Input: part model. Units: mm. Frame: model coordinates. A direction names the side the tool comes from. Give positions to 0.01 mm unless a question says otherwise; leave off trailing zeros. Loops run counter-clockwise (first coordinate to the right, second up) from the corner with the lowest first, then second, coordinate; pieces in that order, holes last. Notation, with made-up numbers: M 75,82.5 L 106,82.5 A6 cw 106,91.5 Z; hole C 83,-1 d3. An arc over 180 degrees is marked long. Answer as a JSON object with one key per item and string values. Group by question number.
1) Draft query along X for faces 1 (the flat face through (18.7, -1, 3)), 2 (the flat face through (14, 8, 0)), 3 (the flat face through (12, 9, -3)), 4 (the flat face through (25.7, 1, 2)). Return one class per face: +X half, -X half, draft (parallel to the pull), parting line (faces both ways), or undercut.
2) Section query A-A on y = 15.75. Return loops of the section in (x, z).
3) Section query B-B on x = 16.75. Return loops of the section in (y, z), plus the area to 4 significant figures.
4) First-contact query: P1, Ø0.9, axis at y = 10.5, z = -1, coming from the +X side; P2, Ø6, axis at x = 15.5, y = 9, coming from the +Z side. Flat tips, straight axial feed; report the tip coordinate or a pass-through.
5) Access query for faces 5 (the flat face through (23.7, 9, -1)), 6 (the flat face through (17.7, 17, -1)), 7 (the flat face through (12.7, -1, 3)), 8 (the flat face through (23.7, 2, 3)). Directions: +Z, -Z, +X, -X, +Y, -Y. A direction counts if a zero-diameter tool reaches every point of the face in a straight line with its end or side. Return the directions, or none.
6) Ray query, L1, parallel to Y at x = 7, z = -1.75; L2, parallel to Y at x = 2.5, z = 2.25; L3, parallel to X at y = 14.75, z = 0.5. Return the intervals inside material, ascending.
7) Section query D-D on z = -2. Return loops of the section in (x, y).
8) Section query C-C on z = 3.25. Return loops of the section in (x, y).
Autodesk Fusion 360 part; units mm, degrees
sketch "Sketch1" plane through (0, 0, 0) normal (0, 0, 1) x (1, 0, 0) in component "case"
  line L0 (0, 0) -> (23.7, 0)
  line L1 (23.7, 0) -> (23.7, 18.6)
  line L2 (23.7, 18.6) -> (0, 18.6)
  line L3 (0, 18.6) -> (0, 0)
  circle A0 centre (21, 16.05) radius 1.5
  circle A1 centre (21, 2.55) radius 1.5
  line L4 (21, 16.05) -> (21, 2.55) construction
  line L5 (23.7, 9.3) -> (0, 9.3) construction
  line L6 (3.75, 0) -> (3.75, 14.85)
  line L7 (3.75, 14.85) -> (17.7, 14.85)
  line L8 (17.7, 14.85) -> (17.7, 18.6)
  line L9 (-2, 21.6) -> (25.7, 21.6)
  line L10 (25.7, 21.6) -> (25.7, -3)
  line L11 (25.7, -3) -> (-2, -3)
  line L12 (-2, -3) -> (-2, 21.6)
  line L13 (11.85, -3) -> (11.85, 21.6) construction
  line L14 (18.7, 0) -> (18.7, -3)
  line L15 (12.7, 0) -> (12.7, -3)
  line L16 (23.7, 14.3) -> (25.7, 14.3)
  line L17 (23.7, 4.3) -> (25.7, 4.3)
  line L18 (24.7, 14.3) -> (24.7, 4.3) construction
  point P0 (21, 9.3)
  point P1 (24.7, 9.3)
  dimension "d1" = 23.7
  dimension "d2" = 18.6
  dimension "d3" = 3
  dimension "d4" = 3
  dimension "d5" = 16.5
  dimension "d6" = 1.2
  dimension "d7" = 6
  dimension "d8" = 3.75
  dimension "d12" = 3
  dimension "d13" = 2
  dimension "d14" = 5
  dimension "d15" = 6
  dimension "d18" = 10
  dimension "d19" = 3.75
extrude "Extrude1" add sketch "Sketch1" against normal blind 3 contours L0 L1 L2 L3 L9 L10 L11 L12 L15 L16 | L0 L1 L2 L6 L7 L8 | L0 L11 L14 L15 | L0 L1 L10 L11 L14 L17 | A0 | A1 in component "case"
extrude "Extrude2" add sketch "Sketch1" along normal blind 6.3 contours L0 L1 L2 L3 L9 L10 L11 L12 L15 L16 | L0 L1 L10 L11 L14 L17 in component "case"
component "case" placed x (1, 0, 0) y (0, 1, 0) z (0, 0, 1) at (0, 0, 0)
equation "d19 = d8"
Output:
{
 "1": {"face 1": "undercut", "face 2": "undercut", "face 3": "draft", "face 4": "+X half"},
 "2": {"outline": "M -2,-3 L 0,-3 L 0,6.3 L -2,6.3 Z; M 17.7,-3 L 25.7,-3 L 25.7,6.3 L 23.7,6.3 L 23.7,0 L 17.7,0 Z"},
 "3": {"outline": "M -3,-3 L 14.85,-3 L 14.85,0 L -3,0 Z; M 18.6,-3 L 21.6,-3 L 21.6,6.3 L 18.6,6.3 Z", "area": "81.45 mm^2"},
 "4": {"P1": "stops at x = 23.7", "P2": "stops at z = 0"},
 "5": {"face 5": "+Z, -Z, +X", "face 6": "+Z, -Z", "face 7": "+Z, -Y", "face 8": "+Z"},
 "6": {"L1": "y = -3 to 14.85, 18.6 to 21.6", "L2": "y = -3 to 0, 18.6 to 21.6", "L3": "x = -2 to 0, 23.7 to 25.7"},
 "7": {"outline": "M -2,-3 L 25.7,-3 L 25.7,4.3 L 23.7,4.3 L 23.7,14.3 L 25.7,14.3 L 25.7,21.6 L -2,21.6 Z; hole M 0,0 L 3.75,0 L 3.75,14.85 L 17.7,14.85 L 17.7,18.6 L 0,18.6 Z"},
 "8": {"outline": "M -2,-3 L 12.7,-3 L 12.7,0 L 0,0 L 0,18.6 L 23.7,18.6 L 23.7,14.3 L 25.7,14.3 L 25.7,21.6 L -2,21.6 Z; M 18.7,-3 L 25.7,-3 L 25.7,4.3 L 23.7,4.3 L 23.7,0 L 18.7,0 Z"}
}
